```python
from build123d import *

# Parameters (mm, degrees)
SKETCH1_W             = 24.62
SKETCH1_H             = 5
SKETCH1_R             = 1.05
BOSS_EXTRUDE1_DEPTH   = 4
SKETCH2_R             = 1.55
BOSS_EXTRUDE2_DEPTH   = 5
BOSS_EXTRUDE2_2_DEPTH = 5
BOSS_EXTRUDE3_DEPTH   = 6.2
BOSS_EXTRUDE4_START   = -6.2
BOSS_EXTRUDE4_DEPTH   = 6.2
CUT_EXTRUDE1_REACH    = 32.969
SKETCH5_W             = 1.45
SKETCH5_H             = 10.45


with BuildPart() as part:
    # Sketch1 → Boss-Extrude1 (new body)
    with BuildSketch(Plane(origin=(0, 0, 0), x_dir=(1, 0, 0), z_dir=(0, 1, 0))):
        with Locations((0, 2.5)):
            Rectangle(SKETCH1_W, SKETCH1_H)
        with Locations(Location((-9.26, 2.95, 0), (0, 0, 270))):
            Circle(SKETCH1_R, mode=Mode.SUBTRACT)
        with Locations(Location((9.26, 2.95, 0), (0, 0, 270))):
            Circle(SKETCH1_R, mode=Mode.SUBTRACT)
    extrude(amount=BOSS_EXTRUDE1_DEPTH)



with BuildPart() as body_2:
    # Sketch2 → Boss-Extrude2 (new body)
    with BuildSketch(Plane(origin=(0, 0, -5), x_dir=(-1, 0, 0), z_dir=(0, 0, -1))):
        Polygon((-12.31, 4), (-12.75, 8.25), (-12.75, 14.45), (-6.55, 14.45), (-6.55, 8.25), (-6.11, 4), align=None)
        with Locations((-9.65, 11.35)):
            Circle(SKETCH2_R, mode=Mode.SUBTRACT)
    extrude(amount=BOSS_EXTRUDE2_DEPTH)


with BuildPart() as body_3:
    # Sketch2 → Boss-Extrude2 2 (new body)
    with BuildSketch(Plane(origin=(0, 0, -5), x_dir=(-1, 0, 0), z_dir=(0, 0, -1))):
        Polygon((6.11, 4), (6.55, 8.25), (6.55, 14.45), (12.75, 14.45), (12.75, 8.25), (12.31, 4), align=None)
        with Locations((9.65, 11.35)):
            Circle(SKETCH2_R, mode=Mode.SUBTRACT)
    extrude(amount=BOSS_EXTRUDE2_2_DEPTH)


with BuildPart() as part_1:
    add(part.part)

    add(body_2.part)  # Boss-Extrude3 merges body 2
    # Sketch6 → Boss-Extrude3 (add)
    with BuildSketch(Plane(origin=(12.31, 0, 0), x_dir=(0, 0, -1), z_dir=(1, 0, 0))):
        with BuildLine():
            Line((5, 0), (5, 4))
            Line((5, 4), (10, 4))
            ThreePointArc((10, 4), (8.201562119, 1.123047352), (5, 0))
        make_face()
    extrude(amount=-BOSS_EXTRUDE3_DEPTH)


    add(body_3.part)  # Boss-Extrude4 merges body 3
    # Sketch7 → Boss-Extrude4 (add)
    with BuildSketch(Plane.ZY.offset(12.31).offset(BOSS_EXTRUDE4_START)):
        with BuildLine():
            Line((-5, 4), (-5, 0))
            ThreePointArc((-5, 0), (-8.201562119, 1.123047352), (-10, 4))
            Line((-10, 4), (-5, 4))
        make_face()
    extrude(amount=BOSS_EXTRUDE4_DEPTH)

    # Cut-Extrude1: up to this face of the body (flat: up to its plane)
    cut_extrude1_end = Plane(part_1.part.faces().sort_by_distance((-12.75, 11.35, -7.5))[0])
    # Sketch5 → Cut-Extrude1 (cut, up to the picked face)
    with BuildSketch(Plane(origin=(12.75, 0, 0), x_dir=(0, 0, -1), z_dir=(1, 0, 0)), mode=Mode.PRIVATE) as cut_extrude1_sk1:
        with Locations((5.725, 9.225)):
            Rectangle(SKETCH5_W, SKETCH5_H)
    cut_extrude1_tool1 = split(extrude(cut_extrude1_sk1.sketch, amount=-CUT_EXTRUDE1_REACH, mode=Mode.PRIVATE), bisect_by=cut_extrude1_end, keep=Keep.BOTH, mode=Mode.PRIVATE)
    add(cut_extrude1_tool1.solids().sort_by(Axis((12.75, 9.225, -5.725), (-1, 0, 0)))[0], mode=Mode.SUBTRACT)


solid = part_1.part
```
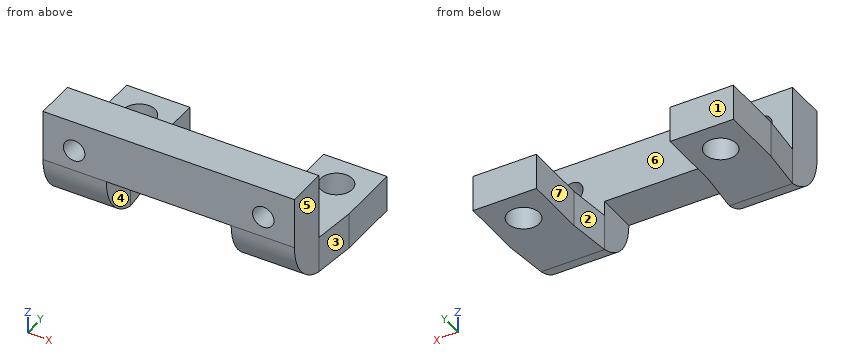
Can you work these out from the model? Positions are in its coordinate system, mm. Face numbers are marked on the shaded views. A direction names the side the tool comes from. Coordinates: 2 decimals unless noted, no trailing zeros. Order: outer loops, then holes, each group sorted by start corner. A loop starts at its lowest first (then second) coordinate and runs counter-clockwise, first axis right, second up.
1. If we section it at C-C (z = -7): Please give me the cut outline in (x, y), then the cut area to 3 significant figures.
2. If we section it at B-B (y = 11.35): Please give me the cut outline in (x, z), then the cut area to 3 significant figures.
3. If we section it at D-D (x = -9): Please give me the cut outline in (y, z) (3 decimals).
4. Thinking about a two-plate mould opening in X: for the marked faces 1, 2 and 3, which applies, +X half, -X half, draft (parallel to the pull), parting line (faces both ways), or undercut?
5. For the marked faces 4, 5, 6 and 7, which set-ups out of +Z, -Z, +X, -X, +Y, -Y let a thin tool reach every point of the face, with its end or its side?
6. If we section it at A-A (z = -2.95): Please give me the cut outline in (x, y).
7. I'm going to push flat-ended pins straight in: pin 1 (1.5 mm diameter, centred on y = 3.5, z = -1.5, fed in from +X); pin 2 (3 mm diameter, centred on y = 6.5, z = -6, fed in from -X); pin 3 (3 mm diameter, centred on y = 1, z = -6, fed in from -X). Where does each tip first touch, or does it pass through?
8. I need wall thicknesses on line 1 (X direction, y = 3.1, z = -2.95); line 2 (X direction, y = 11.35, z = -7.4); line 3 (X direction, y = 9.5, z = -7.5). Which ranges of each line are inside material? Lowest first, please.
Entries:
1. outline: (-12.75, 8.25) - (-12.31, 4) - (-12.31, 0.41) - (-6.11, 0.41) - (-6.11, 4) - (-6.55, 8.25) - (-6.55, 14.45) - (-12.75, 14.45) - close; (6.11, 0.41) - (12.31, 0.41) - (12.31, 4) - (12.75, 8.25) - (12.75, 14.45) - (6.55, 14.45) - (6.55, 8.25) - (6.11, 4) - close; hole circle Ø3.1 at (-9.65, 11.35); hole circle Ø3.1 at (9.65, 11.35)
1. area: 159 mm2
2. outline: (-12.75, -10) - (-11.2, -10) - (-11.2, -6.45) - (-12.75, -6.45) - close; (-8.1, -10) - (-6.55, -10) - (-6.55, -6.45) - (-8.1, -6.45) - close; (6.55, -10) - (8.1, -10) - (8.1, -6.45) - (6.55, -6.45) - close; (11.2, -10) - (12.75, -10) - (12.75, -6.45) - (11.2, -6.45) - close
2. area: 22.0 mm2
3. outline: (0, -5) arc R5.125 ccw to (4, -10) - (9.943, -10) - (9.943, -6.45) - (4, -6.45) - (4, -3.967) - (0, -3.967) - close; (0, -1.933) - (4, -1.933) - (4, 0) - (0, 0) - close; (12.757, -10) - (14.45, -10) - (14.45, -6.45) - (12.757, -6.45) - close
4. face 1: draft
4. face 2: undercut
4. face 3: +X half
5. face 4: -Z, +Y, -Y
5. face 5: +Z, -Z, +X, -Y
5. face 6: +Z, +X, -X, +Y
5. face 7: +Z, -Z, +Y
6. outline: (-12.31, 0) - (-10.31, 0) - (-10.31, 4) - (-12.31, 4) - close; (-8.21, 0) - (8.21, 0) - (8.21, 4) - (-8.21, 4) - close; (10.31, 0) - (12.31, 0) - (12.31, 4) - (10.31, 4) - close
7. pin 1: stops at x = 12.31
7. pin 2: stops at x = -12.72
7. pin 3: stops at x = -12.31
8. line 1: x = -12.31 to -10.31, -8.21 to 8.21, 10.31 to 12.31
8. line 2: x = -12.75 to -11.2, -8.1 to -6.55, 6.55 to 8.1, 11.2 to 12.75
8. line 3: x = -12.75 to -6.55, 6.55 to 12.75
